Here's how the part is built. I have some questions about the finished solid (model axes, mm). Round coordinates to 2 decimals unless told otherwise and drop trailing zeros. Order: outer loops, then holes, each group sorted by start corner. A loop starts at its lowest first (then second) coordinate and runs counter-clockwise, first axis right, second up. Notation, with made-up numbers: (-14, 28) - (-8, 28) arc R16 ccw to (-8, 52) - close; hole circle Ø3 at (53.5, 13). An arc over 180 degrees is marked (long way). Answer as a JSON object with one key per item and string values.
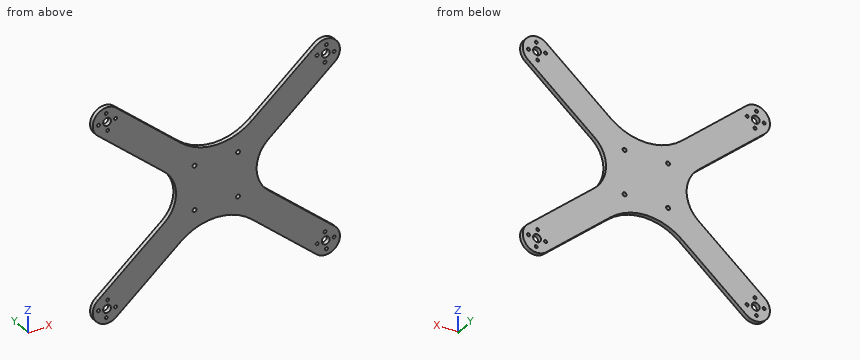
```python
from build123d import *

# Parameters (mm, degrees)
SKETCH2_R           = 1.05
SKETCH2_R_2         = 2.75
BOSS_EXTRUDE2_DEPTH = 3
SKETCH4_R           = 1.375
CUT_EXTRUDE1_DEPTH  = 3


with BuildPart() as part:
    # Sketch2 → Boss-Extrude2 (new body)
    with BuildSketch(Plane(origin=(0, 0, 0), x_dir=(1, 0, 0), z_dir=(0, 1, 0))):
        with BuildLine():
            Line((-83.032320409, 56.618316537), (-36.412926139, 17.5))
            ThreePointArc((-36.412926139, 17.5), (-28.252542121, 0), (-36.412926139, -17.5))
            Line((-36.412926139, -17.5), (-83.032320409, -56.618316537))
            ThreePointArc((-83.032320409, -56.618316537), (-84.264888743, -70.706637066), (-70.176568215, -71.9392054))
            Line((-70.176568215, -71.9392054), (-25, -34.031563673))
            ThreePointArc((-25, -34.031563673), (0, -24.932307816), (25, -34.031563673))
            Line((25, -34.031563673), (70.176568215, -71.9392054))
            ThreePointArc((70.176568215, -71.9392054), (84.264888743, -70.706637066), (83.032320409, -56.618316537))
            Line((83.032320409, -56.618316537), (36.412926139, -17.5))
            ThreePointArc((36.412926139, -17.5), (28.252542121, 0), (36.412926139, 17.5))
            Line((36.412926139, 17.5), (83.032320409, 56.618316537))
            ThreePointArc((83.032320409, 56.618316537), (84.264888743, 70.706637066), (70.176568215, 71.9392054))
            Line((70.176568215, 71.9392054), (25, 34.031563673))
            ThreePointArc((25, 34.031563673), (0, 24.932307816), (-25, 34.031563673))
            Line((-25, 34.031563673), (-70.176568215, 71.9392054))
            ThreePointArc((-70.176568215, 71.9392054), (-84.264888743, 70.706637066), (-83.032320409, 56.618316537))
        make_face()
        with Locations(Location((-77.127378768, 70.255929157, 0), (0, 0, 270))):
            Circle(SKETCH2_R, mode=Mode.SUBTRACT)
        with Locations(Location((-70.627276123, 64.801695425, 0), (0, 0, 270))):
            Circle(SKETCH2_R, mode=Mode.SUBTRACT)
        with Locations(Location((-76.081509855, 58.30159278, 0), (0, 0, 270))):
            Circle(SKETCH2_R, mode=Mode.SUBTRACT)
        with Locations(Location((-82.5816125, 63.755826512, 0), (0, 0, 270))):
            Circle(SKETCH2_R, mode=Mode.SUBTRACT)
        with Locations(Location((-76.604444312, 64.278760969, 0), (0, 0, 270))):
            Circle(SKETCH2_R_2, mode=Mode.SUBTRACT)
        with Locations(Location((-77.127378768, -70.255929157, 0), (0, 0, 90))):
            Circle(SKETCH2_R, mode=Mode.SUBTRACT)
        with Locations(Location((-76.081509855, -58.30159278, 0), (0, 0, 90))):
            Circle(SKETCH2_R, mode=Mode.SUBTRACT)
        with Locations(Location((-82.5816125, -63.755826512, 0), (0, 0, 90))):
            Circle(SKETCH2_R, mode=Mode.SUBTRACT)
        with Locations(Location((-76.604444312, -64.278760969, 0), (0, 0, 90))):
            Circle(SKETCH2_R_2, mode=Mode.SUBTRACT)
        with Locations(Location((-70.627276123, -64.801695425, 0), (0, 0, 90))):
            Circle(SKETCH2_R, mode=Mode.SUBTRACT)
        with Locations(Location((70.627276123, -64.801695425, 0), (0, 0, 270))):
            Circle(SKETCH2_R, mode=Mode.SUBTRACT)
        with Locations(Location((76.604444312, -64.278760969, 0), (0, 0, 270))):
            Circle(SKETCH2_R_2, mode=Mode.SUBTRACT)
        with Locations(Location((82.5816125, -63.755826512, 0), (0, 0, 270))):
            Circle(SKETCH2_R, mode=Mode.SUBTRACT)
        with Locations(Location((76.081509855, -58.30159278, 0), (0, 0, 270))):
            Circle(SKETCH2_R, mode=Mode.SUBTRACT)
        with Locations(Location((77.127378768, -70.255929157, 0), (0, 0, 270))):
            Circle(SKETCH2_R, mode=Mode.SUBTRACT)
        with Locations(Location((76.604444312, 64.278760969, 0), (0, 0, 90))):
            Circle(SKETCH2_R_2, mode=Mode.SUBTRACT)
        with Locations(Location((82.5816125, 63.755826512, 0), (0, 0, 90))):
            Circle(SKETCH2_R, mode=Mode.SUBTRACT)
        with Locations(Location((76.081509855, 58.30159278, 0), (0, 0, 90))):
            Circle(SKETCH2_R, mode=Mode.SUBTRACT)
        with Locations(Location((70.627276123, 64.801695425, 0), (0, 0, 90))):
            Circle(SKETCH2_R, mode=Mode.SUBTRACT)
        with Locations(Location((77.127378768, 70.255929157, 0), (0, 0, 90))):
            Circle(SKETCH2_R, mode=Mode.SUBTRACT)
    extrude(amount=BOSS_EXTRUDE2_DEPTH)

    # Sketch4 → Cut-Extrude1 (cut)
    with BuildSketch(Plane(origin=(0, 0, 0), x_dir=(1, 0, 0), z_dir=(0, 1, 0))):
        with Locations(Location((-15.25, 15.25, 0), (0, 0, 270))):
            Circle(SKETCH4_R)
        with Locations(Location((15.25, -15.25, 0), (0, 0, 270))):
            Circle(SKETCH4_R)
        with Locations(Location((-15.25, -15.25, 0), (0, 0, 270))):
            Circle(SKETCH4_R)
        with Locations(Location((15.25, 15.25, 0), (0, 0, 270))):
            Circle(SKETCH4_R)
    extrude(amount=CUT_EXTRUDE1_DEPTH, mode=Mode.SUBTRACT)


solid = part.part
```
1. Imagine slicing it at C-C (y = 1.2). Give the number of separate pieces and of enclosed holes in the cut face, plus the area to 3 significant figures.
Responses:
{"separate pieces": "1", "enclosed holes": "24", "area": "8,810 mm2"}
2. If I drill on L1, parallel to X at y = 2.5, z = -15.5; L2, parallel to X at y = 1.85, z = 15.25 (3 decimals); L3, parallel to X at y = 0.75, z = 58.5, over which ranges is the centre line in solid material (lowest first)? Write a range as [from, to].
Responses:
{"L1": "[-34.32, -16.6], [-13.9, 13.9], [16.6, 34.32]", "L2": "[-34.088, -16.625], [-13.875, 13.875], [16.625, 34.088]", "L3": "[-84.77, -77.11], [-75.05, -54.16], [54.16, 75.05], [77.11, 84.77]"}
3. For P1, Ø1.5, axis at x = 21.5, y = 1, coming from the +Z side; P2, Ø1, axis at x = 46, y = 0.5, coming from the +Z side; P3, Ø2.5, axis at x = 77.13, z = 70.26, coming from the +Y side; P4, Ø1.5, axis at x = -47, y = 1.5, coming from the +Z side, each with a flat end and sliding along its axis, tell me the tip position at first contact or that it passes through.
Responses:
{"P1": "z = 31.93", "P2": "z = 52.07", "P3": "y = 3", "P4": "z = 53.12"}
4. Imagine slicing it at B-B (z = -27). List the corners of the cut face in (x, y) for me.
Responses:
{"outline": "(-47.73, 0) - (-12.51, 0) - (-12.51, 3) - (-47.73, 3) - close; (12.51, 0) - (47.73, 0) - (47.73, 3) - (12.51, 3) - close"}
5. Imagine slicing it at A-A (x = 54). List the corners of the cut face in (y, z) for me.
Responses:
{"outline": "(0, -58.37) - (3, -58.37) - (3, -32.26) - (0, -32.26) - close; (0, 32.26) - (3, 32.26) - (3, 58.37) - (0, 58.37) - close"}
